For this review, take the finished solid that the model builds, in its own axes (mm). Round coordinates to 2 decimals unless told otherwise and drop trailing zeros. Loops run counter-clockwise (first coordinate to the right, second up) from the corner with the lowest first, then second, coordinate; pieces in that order, holes last.
1. Consider section A-A on z = -18.5. State the section outline as (x, y) points, then the cut area to 3 significant figures.
2. Consider section B-B on y = -6. State the section outline as (x, z) points, then the cut area to 3 significant figures.
3. Clearance check with flat-ended pins moving along their axes: pin 1 Ø2.5 at (x, y) = (-114.3, 0) entering from -Z; pin 2 Ø6.5 at (x, y) = (-63.5, 0) entering from -Z. State where each tip first meets the part, or that it passes through.
4. Consider section D-D on z = 2. State the section outline as (x, y) points, then the cut area to 3 significant figures.
5. Consider section C-C on x = 95.5. State the section outline as (y, z) points, then the cut area to 3 significant figures.
6. To check wall thickness, follow line 1 along X through (y, z) = (-10.9, 0); line 2 along Y through (x, z) = (41, -15.5); line 3 along Y through (x, z) = (-139.7, 24.15). State the ranges of each line that lie inside material, in increasing order.
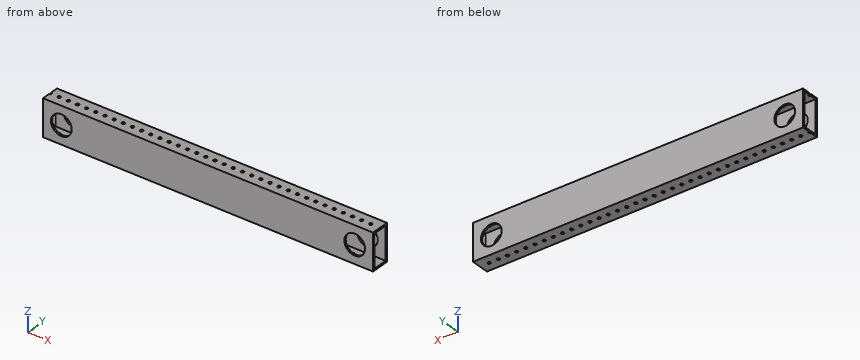
from build123d import *

# Parameters (mm, degrees)
SKETCH1_W           = 50.8
SKETCH1_H           = 25.4
SKETCH1_W_2         = 45.72
SKETCH1_H_2         = 20.32
BOSS_EXTRUDE1_DEPTH = 228.6
SKETCH3_R           = 14.351
CUT_EXTRUDE2_DEPTH  = 232.40501291
SKETCH4_R           = 2.032
CUT_EXTRUDE3_DEPTH  = 235.52055347


with BuildPart() as part:
    # Sketch1 → Boss-Extrude1 (new, symmetric)
    with BuildSketch(Plane(origin=(0, 0, 0), x_dir=(0, 0, -1), z_dir=(1, 0, 0))):
        Rectangle(SKETCH1_W, SKETCH1_H)
        Rectangle(SKETCH1_W_2, SKETCH1_H_2, mode=Mode.SUBTRACT)
    extrude(amount=BOSS_EXTRUDE1_DEPTH, both=True)

    # Sketch3 → Cut-Extrude2 (cut, through all)
    with BuildSketch(Plane.XZ.offset(12.7)):
        with Locations(Location((203.2, 0, 0), (0, 0, 270))):
            Circle(SKETCH3_R)
        with Locations(Location((-203.2, 0, 0), (0, 0, 270))):
            Circle(SKETCH3_R)
    extrude(amount=-CUT_EXTRUDE2_DEPTH, mode=Mode.SUBTRACT)

    # Sketch4 → Cut-Extrude3 (cut, through all)
    with BuildSketch(Plane(origin=(0, 0, -25.4), x_dir=(-1, 0, 0), z_dir=(0, 0, -1))):
        with Locations((-215.9, 0)):
            Circle(SKETCH4_R)
        with Locations((-203.2, 0)):
            Circle(SKETCH4_R)
        with Locations((-190.5, 0)):
            Circle(SKETCH4_R)
        with Locations((-177.8, 0)):
            Circle(SKETCH4_R)
        with Locations((-165.1, 0)):
            Circle(SKETCH4_R)
        with Locations((-152.4, 0)):
            Circle(SKETCH4_R)
        with Locations((-139.7, 0)):
            Circle(SKETCH4_R)
        with Locations((-127, 0)):
            Circle(SKETCH4_R)
        with Locations((-114.3, 0)):
            Circle(SKETCH4_R)
        with Locations((-101.6, 0)):
            Circle(SKETCH4_R)
        with Locations((-88.9, 0)):
            Circle(SKETCH4_R)
        with Locations((-76.2, 0)):
            Circle(SKETCH4_R)
        with Locations((-63.5, 0)):
            Circle(SKETCH4_R)
        with Locations((-50.8, 0)):
            Circle(SKETCH4_R)
        with Locations((-38.1, 0)):
            Circle(SKETCH4_R)
        with Locations((-25.4, 0)):
            Circle(SKETCH4_R)
        with Locations((-12.7, 0)):
            Circle(SKETCH4_R)
        Circle(SKETCH4_R)
        with Locations((12.7, 0)):
            Circle(SKETCH4_R)
        with Locations((25.4, 0)):
            Circle(SKETCH4_R)
        with Locations((38.1, 0)):
            Circle(SKETCH4_R)
        with Locations((50.8, 0)):
            Circle(SKETCH4_R)
        with Locations((63.5, 0)):
            Circle(SKETCH4_R)
        with Locations((76.2, 0)):
            Circle(SKETCH4_R)
        with Locations((88.9, 0)):
            Circle(SKETCH4_R)
        with Locations((101.6, 0)):
            Circle(SKETCH4_R)
        with Locations((114.3, 0)):
            Circle(SKETCH4_R)
        with Locations((127, 0)):
            Circle(SKETCH4_R)
        with Locations((139.7, 0)):
            Circle(SKETCH4_R)
        with Locations((152.4, 0)):
            Circle(SKETCH4_R)
        with Locations((165.1, 0)):
            Circle(SKETCH4_R)
        with Locations((177.8, 0)):
            Circle(SKETCH4_R)
        with Locations((190.5, 0)):
            Circle(SKETCH4_R)
        with Locations((203.2, 0)):
            Circle(SKETCH4_R)
        with Locations((215.9, 0)):
            Circle(SKETCH4_R)
        with Locations((228.6, 0)):
            Circle(SKETCH4_R)
    extrude(amount=-CUT_EXTRUDE3_DEPTH, mode=Mode.SUBTRACT)


solid = part.part
Resolved:
1. outline: (-228.6, -12.7) - (228.6, -12.7) - (228.6, -10.16) - (-228.6, -10.16) - close; (-228.6, 10.16) - (228.6, 10.16) - (228.6, 12.7) - (-228.6, 12.7) - close
1. area: 2,320 mm2
2. outline: (-228.6, -25.4) - (228.6, -25.4) - (228.6, -22.86) - (-228.6, -22.86) - close; (-228.6, 22.86) - (228.6, 22.86) - (228.6, 25.4) - (-228.6, 25.4) - close
2. area: 2,320 mm2
3. pin 1: passes through
3. pin 2: stops at z = -25.4
4. outline: (-228.6, -12.7) - (-217.41, -12.7) - (-217.41, -10.16) - (-228.6, -10.16) - close; (-228.6, 10.16) - (-217.41, 10.16) - (-217.41, 12.7) - (-228.6, 12.7) - close; (-188.99, -12.7) - (188.99, -12.7) - (188.99, -10.16) - (-188.99, -10.16) - close; (-188.99, 10.16) - (188.99, 10.16) - (188.99, 12.7) - (-188.99, 12.7) - close; (217.41, -12.7) - (228.6, -12.7) - (228.6, -10.16) - (217.41, -10.16) - close; (217.41, 10.16) - (228.6, 10.16) - (228.6, 12.7) - (217.41, 12.7) - close
4. area: 2,030 mm2
5. outline: (-12.7, -25.4) - (12.7, -25.4) - (12.7, 25.4) - (-12.7, 25.4) - close; hole (-10.16, -22.86) - (10.16, -22.86) - (10.16, 22.86) - (-10.16, 22.86) - close
5. area: 361 mm2
6. line 1: x = -228.6 to -217.55, -188.85 to 188.85, 217.55 to 228.6
6. line 2: y = -12.7 to -10.16, 10.16 to 12.7
6. line 3: y = -12.7 to -2.03, 2.03 to 12.7
